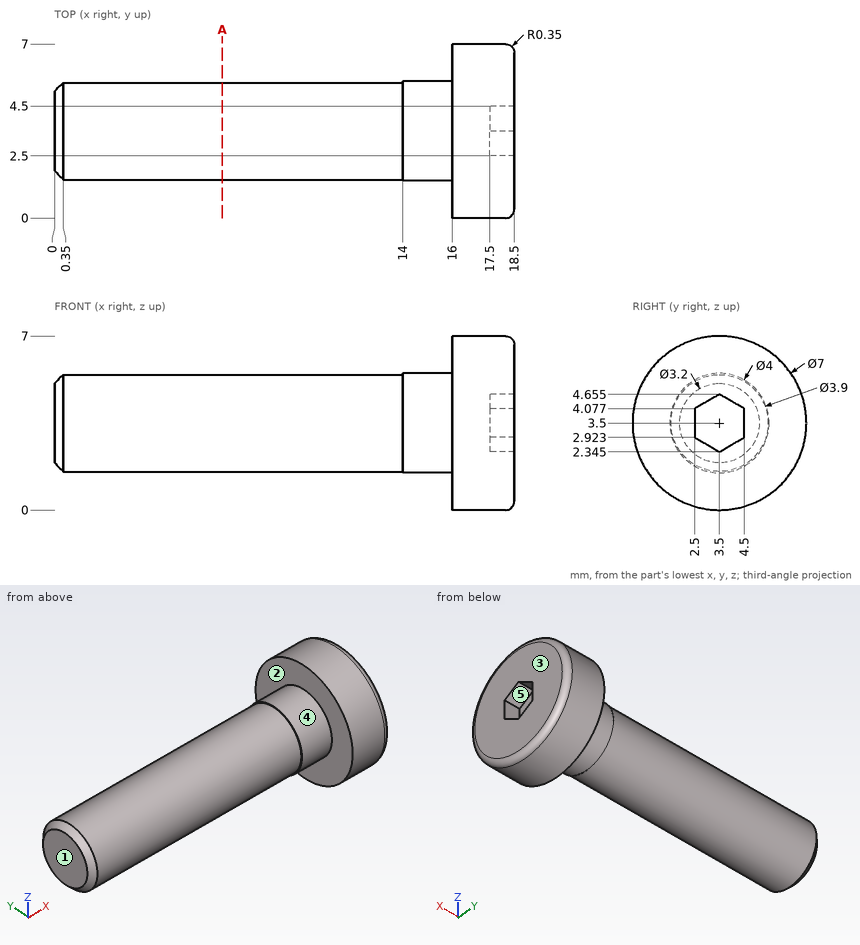
The drawing under review shows one solid part. Ordinate dimensions are in mm from its lowest x, y, z. A direction names the side the tool comes from. Give positions to 0.01 mm unless a question says otherwise; leave off trailing zeros. Write each loop counter-clockwise with the first axis right and the second up, starting at its lowest first coordinate (ties: lowest second). Pieces come first, ordered by that corner, then holes.
1. Draft analysis for pull direction Y (two halves, no side actions). For the marked faces 3, 4 and 5, state which applies: +Y half, -Y half, draft (parallel to the pull), parting line (faces both ways), or undercut.
2. Wall thickness on L1, parallel to X at y = 1.5, z = 4.25; L2, parallel to Z at x = 1.5, y = 5.25; L3, parallel to Y at x = 3.25, z = 3 (1 decimal): over which ranges is each line inside the solid? List them lowest first.
3. For P1, Ø4, axis at x = 4, y = 3, coming from the +Z side; P2, Ø2, axis at x = 11, z = 2.5, coming from the -Y side, all flat-tipped, find the tip position at first contact; note any pin that passes through.
4. Add section A-A, the plane x = 6.75. Write out the cut boundary in (y, z).
5. Tool access review of the marked faces 1 and 2: name each direction out of +Z, -Z, +X, -X, +Y, -Y from which nothing blocks a thin tool from reaching the whole face with its end or side.
Worked answers:
1. face 3: draft
1. face 4: parting line
1. face 5: undercut
2. L1: x = 16 to 18.5
2. L2: z = 2.64 to 4.36
2. L3: y = 1.6 to 5.4
3. P1: stops at z = 5.45
3. P2: stops at y = 1.55
4. outline: circle Ø3.9 at (3.5, 3.5)
5. face 1: +Z, -Z, -X, +Y, -Y
5. face 2: -X
